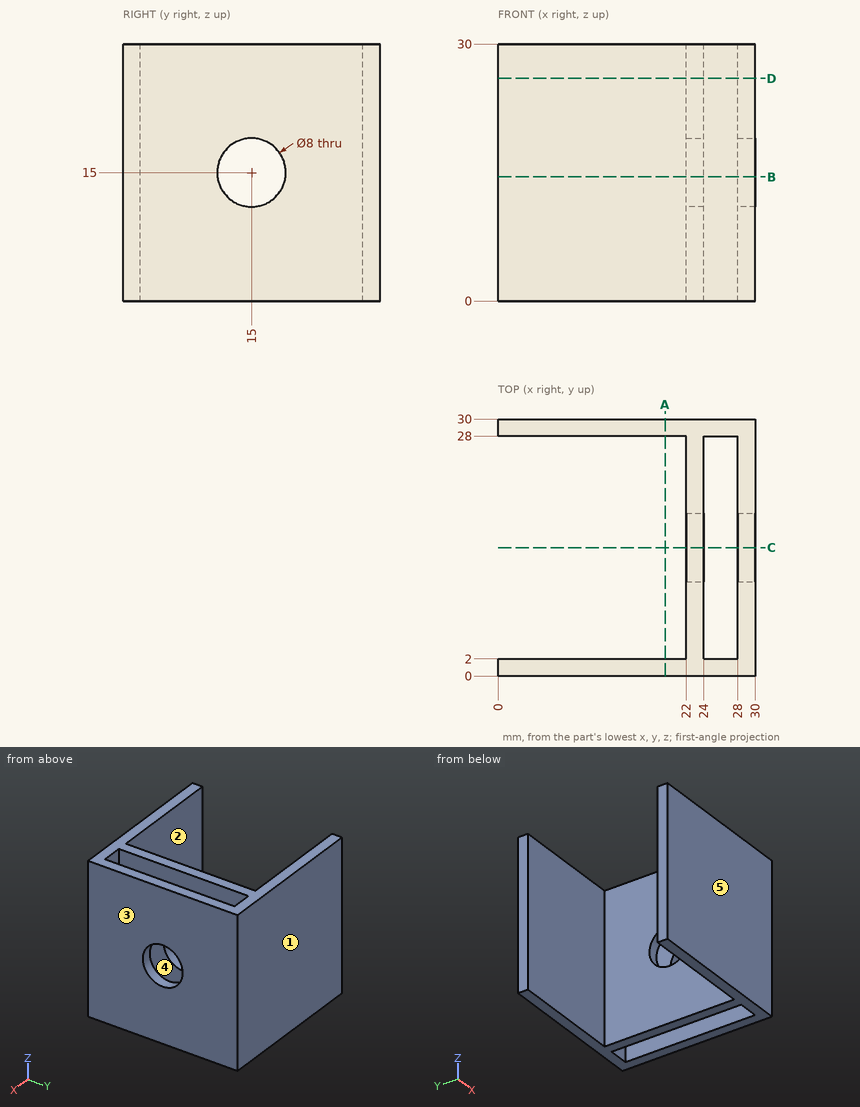
Geometry: see drawing. Coordinates: mm, zero at the bounding-box minimum. A direction names the side the tool comes from. Coordinates: 2 decimals unless noted, no trailing zeros. Order: outer loops, then holes, each group sorted by start corner. A loop starts at its lowest first (then second) coordinate and runs counter-clockwise, first axis right, second up. Notation, with made-up numbers: (48.5, 11) -> (79.5, 11) arc R21 ccw to (79.5, 16) -> close; hole circle Ø3 at (-17, -16.5). An arc over 180 degrees is marked (long way). Write each question's results on one line, items separated by ' | '. Start each with the question number.
1) First-contact query: pin 1 (13 mm diameter, centred on y = 15.5, z = 9, fed in from -X). Flat tip, straight axial feed; report the tip coordinate or a pass-through.
2) Cut plane B-B, the plane z = 14.5. Output: boundary loops of the cut face in (x, y), and give its area (3 significant figures).
3) Cut plane A-A, the plane x = 19.5. Output: boundary loops of the cut face in (y, z).
4) Mould query, pull axis Y, two halves, no side actions, for the marked faces 3, 4 and 5. Classes: released by +Y, released by -Y, zero draft, split by the parting line, or undercut.
5) Material intervals for line 1 along Y through (x, z) = (25.25, 17); line 2 along Y through (x, z) = (29.1, 15); line 3 along X through (y, z) = (18, 10.75), sorted ascending.
6) Cut plane D-D, the plane z = 26. Output: boundary loops of the cut face in (x, y).
7) Cut plane C-C, the plane y = 15. Output: boundary loops of the cut face in (x, z).
8) Set-up query: the marked faces 1 and 2. Return all of +Z, -Z, +X, -X, +Y, -Y with unobstructed straight access to the full face (end or side cutting, diameter ignored); none if empty.
Checks:
1) pin 1: x = 22
2) outline: (0, 0) -> (30, 0) -> (30, 11.03) -> (28, 11.03) -> (28, 2) -> (24, 2) -> (24, 11.03) -> (22, 11.03) -> (22, 2) -> (0, 2) -> close; (0, 28) -> (22, 28) -> (22, 18.97) -> (24, 18.97) -> (24, 28) -> (28, 28) -> (28, 18.97) -> (30, 18.97) -> (30, 30) -> (0, 30) -> close | area: 192 mm^2
3) outline: (0, 0) -> (2, 0) -> (2, 30) -> (0, 30) -> close; (28, 0) -> (30, 0) -> (30, 30) -> (28, 30) -> close
4) face 3: zero draft | face 4: undercut | face 5: released by -Y
5) line 1: 0 to 2, 28 to 30 | line 2: 0 to 11, 19 to 30 | line 3: 22 to 24, 28 to 30
6) outline: (0, 0) -> (30, 0) -> (30, 30) -> (0, 30) -> (0, 28) -> (22, 28) -> (22, 2) -> (0, 2) -> close; hole (24, 2) -> (28, 2) -> (28, 28) -> (24, 28) -> close
7) outline: (22, 0) -> (24, 0) -> (24, 11) -> (22, 11) -> close; (22, 19) -> (24, 19) -> (24, 30) -> (22, 30) -> close; (28, 0) -> (30, 0) -> (30, 11) -> (28, 11) -> close; (28, 19) -> (30, 19) -> (30, 30) -> (28, 30) -> close
8) face 1: +Z, -Z, +X, -X, +Y | face 2: +Z, -Z, -X
